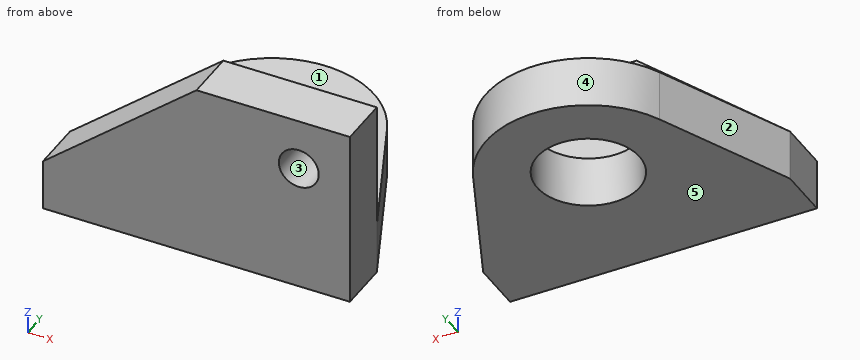
Autodesk Inventor part; units mm, degrees
ref_plane "YZ Plane" through (0, 0, 0) normal (1, 0, 0) x (0, 1, 0)
ref_plane "XZ Plane" through (0, 0, 0) normal (0, 1, 0) x (-1, 0, 0)
ref_plane "XY Plane" through (0, 0, 0) normal (0, 0, 1) x (1, 0, 0)
sketch "Sketch1" plane through (0, 0, 0) normal (0, 1, 0) x (-1, 0, 0)
  line L0 (0, 0) -> (38.1, 0)
  line L1 (38.1, 0) -> (38.1, -19.05)
  line L2 (38.1, -19.05) -> (0, -19.05)
  line L3 (0, -19.05) -> (0, 0)
  circle A0 centre (6.35, -3.175) radius 2.4765
  circle A1 centre (31.75, -3.175) radius 2.4765
  dimension "d0" = 4.953
  dimension "d1" = 4.953
  dimension "d2" = 25.4
  dimension "d3" = 6.35
  dimension "d4" = 3.175
  dimension "d5" = 6.35
  dimension "d6" = 19.05
extrude "Extrusion1" add sketch "Sketch1" along normal blind 6.35
sketch "Sketch2" plane through (0, 0, -19.05) normal (0, 0, -1) x (-1, 0, 0)
  line L0 (38.1, 0) -> (0, 0)
  line L1 (38.1, 0) -> (38.1, 6.35)
  line L2 (0, 6.35) -> (38.1, 6.35)
  line L3 (0, 0) -> (0, 6.35)
  circle A0 centre (19.05, 17.7546) radius 14.2748
  circle A1 centre (19.05, 17.7546) radius 6.35
  line L4 (38.1, 6.35) -> (0, 6.35)
  line L5 (0, 6.35) -> (7.4663, 22.9612)
  line L6 (38.1, 6.35) -> (30.6337, 22.9612)
  arc A2 (30.6337, 22.9612) -> (7.4663, 22.9612) centre (19.05, 17.7546) ccw
  point P0 (0, 0)
  dimension "d9" = 6.35
  dimension "d10" = 12.7
extrude "Extrusion2" add sketch "Sketch2" against normal blind 6.35 contours L2 A0 L6 | L5 A0 L2 | L2 A0 L5 A2 L6
sketch "Sketch3" plane through (-38.1, 0, 0) normal (0, 0, 1) x (1, 0, 0)
  line L0 (38.1, 0) -> (0, 0)
  line L1 (38.1, 0) -> (38.1, 6.35)
  line L2 (0, 6.35) -> (38.1, 6.35)
  line L3 (0, 0) -> (0, 6.35)
extrude "Extrusion3" add sketch "Sketch3" along normal blind 3.175
sketch "Sketch4" plane through (0, 6.35, 0) normal (0, 1, 0) x (1, 0, 0)
  line L0 (0, 12.7) -> (-38.1, 12.7)
  line L1 (-38.1, 12.7) -> (-38.1, -3.175)
  line L2 (0, -3.175) -> (-38.1, -3.175)
  line L3 (0, 12.7) -> (0, -3.175)
  circle A0 centre (-6.35, 3.175) radius 2.4765
  circle A1 centre (-31.75, 3.175) radius 2.4765
  line L4 (-38.1, 12.7) -> (-19.05, -3.175)
  line L5 (-38.1, -3.175) -> (0, -3.175)
  point P0 (0, 0)
extrude "Extrusion4" cut sketch "Sketch4" against normal blind 25.4 contours L4 L2 L1
equation "\"d5\" = d3"
properties part number "Encoder mount_left"
Can you work these out from the model? Positions are in its coordinate system, mm. Face numbers are marked on the shaded views. A direction names the side the tool comes from. Coordinates: 2 decimals unless noted, no trailing zeros. Loops run counter-clockwise (first coordinate to the right, second up) from the corner with the lowest first, then second, coordinate; pieces in that order, holes last. Notation, with made-up numbers: (-20, 49.5) - (7, 49.5) arc R34 cw to (7, 84.5) - close; hole circle Ø1 at (61.5, -4.75). An arc over 180 degrees is marked (long way). Answer as a JSON object with one key per item and string values. Group by question number.
Item 1: If we section it at D-D (z = -17.25): List the corners of the cut face in (x, y) for me.
Item 2: If I drill on L1, parallel to Y at x = -19.05, z = -16; L2, parallel to Z at x = -13.5, y = 28.5; L3, parallel to Z at x = -6, y = 3 (3 decimals), over which ranges is the centre line in solid material (lowest first)? Write a range as from..to.
Item 3: For pin 1 (6 mm diameter, centred on x = -10.5, y = 14, fed in from +Z); pin 2 (5 mm diameter, centred on x = -27, z = -7, fed in from +Y); pin 3 (6 mm diameter, centred on x = -27, y = 5, fed in from +Z), each with a flat end and sliding along its axis, tell me the tip position at first contact or that it passes through.
Item 4: On a 3-axis mill with a long thin cutter (end or side, diameter ignored), from which of +Z, -Z, +X, -X, +Y, -Y can I reach the whole of each face in a straight line? I mean the marked faces 1 and 2. Say none if no direction works.
Item 5: If we mould it in two halves opening along Z, with no side actions, what happens to the marked faces 3, 4 and 5? For each: released by +Z, released by -Z, zero draft, split by the parting line, or undercut.
Item 6: If we section it at C-C (y = 16): List the corners of the cut face in (x, z) for me, plus the area to 3 significant figures.
Item 7: If we section it at A-A (z = -3.75): List the corners of the cut face in (x, y) for me.
Item 8: If we section it at B-B (x = -4.5): List the corners of the cut face in (y, z) for me (3 decimals), plus the area to 3 significant figures.
Returned:
{
 "1": {"outline": "(-38.1, 0) - (0, 0) - (0, 6.35) - (-7.47, 22.96) arc R12.7 ccw to (-30.63, 22.96) - (-38.1, 6.35) - close; hole circle Ø12.7 at (-19.05, 17.75)"},
 "2": {"L1": "y = 0..11.4, 24.1..30.45", "L2": "z = -19.05..-12.7", "L3": "z = -19.05..-5.627, -0.723..3.175"},
 "3": {"pin 1": "stops at z = -12.7", "pin 2": "stops at y = 6.35", "pin 3": "stops at z = -0.95"},
 "4": {"face 1": "+Z, +X, -X, +Y", "face 2": "+Z, -Z, -X, +Y"},
 "5": {"face 3": "undercut", "face 4": "zero draft", "face 5": "released by -Z"},
 "6": {"outline": "(-33.76, -19.05) - (-25.15, -19.05) - (-25.15, -12.7) - (-33.76, -12.7) - close; (-12.95, -19.05) - (-4.34, -19.05) - (-4.34, -12.7) - (-12.95, -12.7) - close", "area": "109 mm²"},
 "7": {"outline": "(-27.36, 0) - (-8.76, 0) - (-8.76, 6.35) - (-27.36, 6.35) - close; (-3.94, 0) - (0, 0) - (0, 6.35) - (-3.94, 6.35) - close"},
 "8": {"outline": "(0, -19.05) - (16.362, -19.05) - (16.362, -12.7) - (6.35, -12.7) - (6.35, -4.821) - (0, -4.821) - close; (0, -1.529) - (6.35, -1.529) - (6.35, 3.175) - (0, 3.175) - close", "area": "184 mm²"}
}
